Input: part model. Units: mm. Frame: model coordinates. Face numbers are marked on the shaded views. A direction names the side the tool comes from. Coordinates: 2 decimals unless noted, no trailing zeros. Order: outer loops, then holes, each group sorted by start corner. A loop starts at its lowest first (then second) coordinate and runs counter-clockwise, first axis right, second up. Notation, with made-up numbers: (-17.75, 27) - (22.25, 27) arc R19 ccw to (22.25, 38) - close; hole circle Ø8 at (-13.5, -9). An arc over 180 degrees is marked (long way). One line per question, with ' | ' between items.
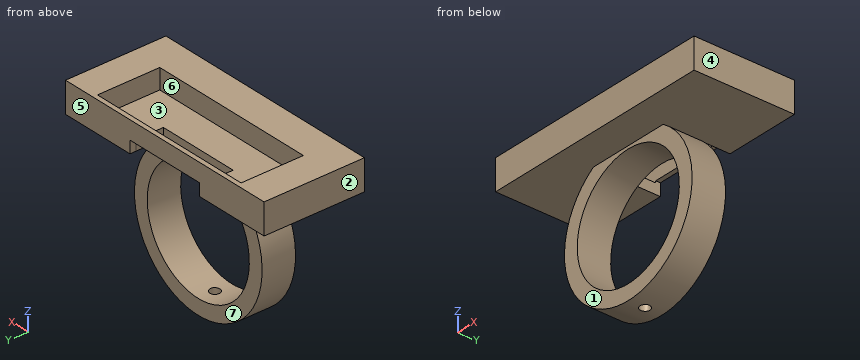
from build123d import *

# Parameters (mm, degrees)
CROQUIS1_R                   = 22.5
CROQUIS1_R_2                 = 18
SALIENTE_EXTRUIR1_DEPTH      = 10
SALIENTE_EXTRUIR2_DEPTH      = 10
SALIENTE_EXTRUIR2_DEPTH_BACK = 20
CROQUIS3_W                   = 70
CROQUIS3_H                   = 9.106451256
CROQUIS5_R                   = 1.5
CORTAR_EXTRUIR1_DEPTH        = 50.053642187
CROQUIS7_W                   = 50
CROQUIS7_H                   = 10.485407271
CORTAR_EXTRUIR2_DEPTH        = 5
CROQUIS8_W                   = 50.630312491
CROQUIS8_H                   = 6
CORTAR_EXTRUIR3_DEPTH        = 20
CROQUIS11_W                  = 24.591659355
CROQUIS11_H                  = 8.221287074
CORTAR_EXTRUIR4_DEPTH        = 16
CROQUIS12_W                  = 6
CROQUIS12_H                  = 1.38614326
SALIENTE_EXTRUIR3_DEPTH      = 56
CROQUIS13_W                  = 24.583761772
CROQUIS13_H                  = 3.662244936
CORTAR_EXTRUIR5_DEPTH        = 5


with BuildPart() as part:
    # Croquis1 → Saliente-Extruir1 (new body)
    with BuildSketch(Plane(origin=(0, 0, 0), x_dir=(1, 0, 0), z_dir=(0, 1, 0))):
        with Locations(Location((0, 0, 0), (0, 0, 270))):
            Circle(CROQUIS1_R)
        with Locations(Location((0, 0, 0), (0, 0, 270))):
            Circle(CROQUIS1_R_2, mode=Mode.SUBTRACT)
    extrude(amount=SALIENTE_EXTRUIR1_DEPTH)

    # Croquis3 → Saliente-Extruir2 (add, two sides: drawn at the far end of the back side and taken through both)
    with BuildSketch(Plane(origin=(0, 10, 0), x_dir=(1, 0, 0), z_dir=(0, 1, 0)).offset(-SALIENTE_EXTRUIR2_DEPTH_BACK)):
        with Locations((0, -23.39779961)):
            Rectangle(CROQUIS3_W, CROQUIS3_H)
    extrude(amount=SALIENTE_EXTRUIR2_DEPTH + SALIENTE_EXTRUIR2_DEPTH_BACK)

    # Croquis5 → Cortar-Extruir1 (cut, through all)
    with BuildSketch(Plane.XY):
        with Locations(Location((0, 5, 0), (0, 0, 90))):
            Circle(CROQUIS5_R)
    extrude(amount=-CORTAR_EXTRUIR1_DEPTH, mode=Mode.SUBTRACT)

    # Croquis7 → Cortar-Extruir2 (cut)
    with BuildSketch(Plane.XY.offset(27.951025238)):
        with Locations((0, 6.110348598)):
            Rectangle(CROQUIS7_W, CROQUIS7_H)
    extrude(amount=-CORTAR_EXTRUIR2_DEPTH, mode=Mode.SUBTRACT)

    # Croquis8 → Cortar-Extruir3 (cut)
    with BuildSketch(Plane(origin=(0, 20, 0), x_dir=(1, 0, 0), z_dir=(0, 1, 0))):
        with Locations((0.058181837, -24.951025238)):
            Rectangle(CROQUIS8_W, CROQUIS8_H)
    extrude(amount=-CORTAR_EXTRUIR3_DEPTH, mode=Mode.SUBTRACT)

    # Croquis11 → Cortar-Extruir4 (cut)
    with BuildSketch(Plane(origin=(0, 0, 18.844573982), x_dir=(-1, 0, 0), z_dir=(0, 0, -1))):
        with Locations((0.00225284, 14.110643537)):
            Rectangle(CROQUIS11_W, CROQUIS11_H)
    extrude(amount=-CORTAR_EXTRUIR4_DEPTH, mode=Mode.SUBTRACT)

    # Croquis12 → Saliente-Extruir3 (add)
    with BuildSketch(Plane.ZY.offset(-25.373338083)):
        with Locations((24.951025238, 19.30692837)):
            Rectangle(CROQUIS12_W, CROQUIS12_H)
    extrude(amount=SALIENTE_EXTRUIR3_DEPTH)

    # Croquis13 → Cortar-Extruir5 (cut)
    with BuildSketch(Plane(origin=(0, 20, 0), x_dir=(1, 0, 0), z_dir=(0, 1, 0))):
        with Locations((-0.006201632, -20.67569645)):
            Rectangle(CROQUIS13_W, CROQUIS13_H)
    extrude(amount=-CORTAR_EXTRUIR5_DEPTH, mode=Mode.SUBTRACT)


solid = part.part
Item 1: Section B-B on x = 0. Return the cut outline in (y, z), and give its area (3 significant figures).
Data:
outline: (-10, 18.84) - (0, 18.84) - (0, 18) - (10, 18) - (10, 21.95) - (0, 21.95) - (0, 27.95) - (-10, 27.95) - close; (0, -22.5) - (3.5, -22.5) - (3.5, -18) - (0, -18) - close; (6.5, -22.5) - (10, -22.5) - (10, -18) - (6.5, -18) - close; (18.61, 22.51) - (20, 22.51) - (20, 27.95) - (18.61, 27.95) - close | area: 170 mm^2
Item 2: Section A-A on z = 0. Return the cut outline in (x, y).
Data:
outline: (-22.5, 0) - (-18, 0) - (-18, 10) - (-22.5, 10) - close; (18, 0) - (22.5, 0) - (22.5, 10) - (18, 10) - close
Item 3: Contact query for flat-ended pins moving along their axis: P1, Ø20.5, axis at x = -10, z = 3, coming from the -Y side; P2, Ø6, axis at x = -2.5, y = 11.5, coming from the -Z side; P3, Ø0.7, axis at x = 2.5, y = 19.5, coming from the -Z side. Output: stop coordinate, or through.
Data:
P1: y = 0 | P2: z = -22.5 | P3: z = 22.51
Item 4: Draft query along X for the marked faces 1, 2, 3 and 4. Return one class per face: released by +X, released by -X, zero draft, split by the parting line, or undercut.
Data:
face 1: zero draft | face 2: released by -X | face 3: undercut | face 4: released by +X
Item 5: Ray query, line 1 (Z direction, x = 14.5, y = 8.25); line 2 (X direction, y = 4, z = 0); line 3 (Z direction, x = 11, y = -4.5). Return the intervals inside material, ascending.
Data:
line 1: -17.2 to -10.67, 10.67 to 17.2, 18.84 to 21.95 | line 2: -22.5 to -18, 18 to 22.5 | line 3: 18.84 to 27.95
Item 6: Section D-D on x = 29.5. Return the cut outline in (y, z).
Data:
outline: (-10, 18.84) - (20, 18.84) - (20, 27.95) - (-10, 27.95) - close
Item 7: Access query for the marked faces 5, 6 and 7. Directions: +Z, -Z, +X, -X, +Y, -Y. A direction counts if a zero-diameter tool reaches every point of the face in a straight line with its end or side. Return the directions, or none.
Data:
face 5: +Z, -Z, +X, -X, +Y | face 6: +Z | face 7: -Z, +Y
Item 8: Section C-C on y = 8. Return the cut outline in (x, z), and give its area (3 significant figures).
Data:
outline: (-35, 18.84) - (-12.29, 18.84) arc R22.5 ccw (long way) to (12.29, 18.84) - (35, 18.84) - (35, 27.95) - (25.37, 27.95) - (25.37, 21.95) - (-25.26, 21.95) - (-25.26, 27.95) - (-35, 27.95) - close; hole circle Ø36 at (0, 0) | area: 845 mm^2
